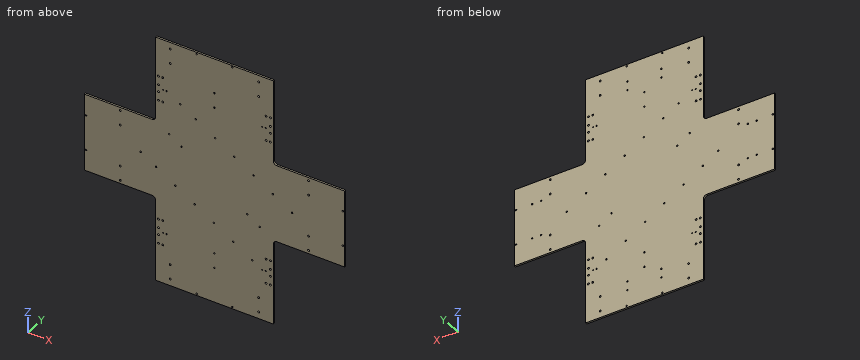
from build123d import *

# Parameters (mm, degrees)
BOSS_EXTRUDE1_DEPTH = 5
SKETCH2_R           = 2.125
CUT_EXTRUDE1_DEPTH  = 3
SKETCH4_R           = 2.6
SKETCH4_R_2         = 1.6
CUT_EXTRUDE3_DEPTH  = 10
SKETCH5_R           = 2.125
CUT_EXTRUDE4_DEPTH  = 10
FILLET1_R           = 10
SKETCH6_R           = 2.6
CUT_EXTRUDE5_DEPTH  = 10
SKETCH7_R           = 2.125
CUT_EXTRUDE6_DEPTH  = 10
SKETCH8_R           = 2.1
CUT_EXTRUDE7_DEPTH  = 10


with BuildPart() as part:
    # Sketch1 → Boss-Extrude1 (new body)
    with BuildSketch(Plane(origin=(0, 0, 0), x_dir=(1, 0, 0), z_dir=(0, 1, 0))):
        Polygon((165, 352), (-165, 352), (-165, 110), (-365, 110), (-365, -110), (-165, -110), (-165, -352), (165, -352), (165, -110), (365, -110), (365, 110), (165, 110), align=None)
    extrude(amount=BOSS_EXTRUDE1_DEPTH)

    # Sketch2 → Cut-Extrude1 (cut)
    with BuildSketch(Plane(origin=(0, 5, 0), x_dir=(1, 0, 0), z_dir=(0, 1, 0))):
        with Locations(Location((315, 49.5, 0), (0, 0, 270))):
            Circle(SKETCH2_R)
        with Locations(Location((290, 49.5, 0), (0, 0, 270))):
            Circle(SKETCH2_R)
        with Locations(Location((290, -49.5, 0), (0, 0, 90))):
            Circle(SKETCH2_R)
        with Locations(Location((315, -49.5, 0), (0, 0, 90))):
            Circle(SKETCH2_R)
        with Locations(Location((-315, -49.5, 0), (0, 0, 270))):
            Circle(SKETCH2_R)
        with Locations(Location((-290, -49.5, 0), (0, 0, 270))):
            Circle(SKETCH2_R)
        with Locations(Location((-290, 49.5, 0), (0, 0, 90))):
            Circle(SKETCH2_R)
        with Locations(Location((-315, 49.5, 0), (0, 0, 90))):
            Circle(SKETCH2_R)
        with Locations(Location((47.5, 302, 0), (0, 0, 270))):
            Circle(SKETCH2_R)
        with Locations(Location((47.5, 277, 0), (0, 0, 270))):
            Circle(SKETCH2_R)
        with Locations(Location((-47.5, 277, 0), (0, 0, 90))):
            Circle(SKETCH2_R)
        with Locations(Location((-47.5, 302, 0), (0, 0, 90))):
            Circle(SKETCH2_R)
        with Locations(Location((-47.5, -302, 0), (0, 0, 270))):
            Circle(SKETCH2_R)
        with Locations(Location((-47.5, -277, 0), (0, 0, 270))):
            Circle(SKETCH2_R)
        with Locations(Location((47.5, -277, 0), (0, 0, 90))):
            Circle(SKETCH2_R)
        with Locations(Location((47.5, -302, 0), (0, 0, 90))):
            Circle(SKETCH2_R)
    extrude(amount=-CUT_EXTRUDE1_DEPTH, mode=Mode.SUBTRACT)

    # Sketch4 → Cut-Extrude3 (cut)
    with BuildSketch(Plane(origin=(0, 5, 0), x_dir=(1, 0, 0), z_dir=(0, 1, 0))):
        with Locations(Location((-157, 172, 0), (0, 0, 270))):
            Circle(SKETCH4_R)
        with Locations(Location((-145, 172, 0), (0, 0, 270))):
            Circle(SKETCH4_R)
        with Locations(Location((-157, 197, 0), (0, 0, 270))):
            Circle(SKETCH4_R)
        with Locations(Location((-157, 217, 0), (0, 0, 270))):
            Circle(SKETCH4_R)
        with Locations(Location((-157, 242, 0), (0, 0, 270))):
            Circle(SKETCH4_R)
        with Locations(Location((-145, 242, 0), (0, 0, 270))):
            Circle(SKETCH4_R)
        with Locations(Location((145, 242, 0), (0, 0, 90))):
            Circle(SKETCH4_R)
        with Locations(Location((157, 242, 0), (0, 0, 90))):
            Circle(SKETCH4_R)
        with Locations(Location((157, 217, 0), (0, 0, 90))):
            Circle(SKETCH4_R)
        with Locations(Location((157, 197, 0), (0, 0, 90))):
            Circle(SKETCH4_R)
        with Locations(Location((145, 172, 0), (0, 0, 90))):
            Circle(SKETCH4_R)
        with Locations(Location((157, 172, 0), (0, 0, 90))):
            Circle(SKETCH4_R)
        with Locations(Location((157, -172, 0), (0, 0, 270))):
            Circle(SKETCH4_R)
        with Locations(Location((145, -172, 0), (0, 0, 270))):
            Circle(SKETCH4_R)
        with Locations(Location((157, -197, 0), (0, 0, 270))):
            Circle(SKETCH4_R)
        with Locations(Location((157, -217, 0), (0, 0, 270))):
            Circle(SKETCH4_R)
        with Locations(Location((157, -242, 0), (0, 0, 270))):
            Circle(SKETCH4_R)
        with Locations(Location((145, -242, 0), (0, 0, 270))):
            Circle(SKETCH4_R)
        with Locations(Location((-145, -242, 0), (0, 0, 90))):
            Circle(SKETCH4_R)
        with Locations(Location((-157, -242, 0), (0, 0, 90))):
            Circle(SKETCH4_R)
        with Locations(Location((-157, -217, 0), (0, 0, 90))):
            Circle(SKETCH4_R)
        with Locations(Location((-157, -197, 0), (0, 0, 90))):
            Circle(SKETCH4_R)
        with Locations(Location((-145, -172, 0), (0, 0, 90))):
            Circle(SKETCH4_R)
        with Locations(Location((-157, -172, 0), (0, 0, 90))):
            Circle(SKETCH4_R)
        with Locations(Location((144, -207, 0), (0, 0, 270))):
            Circle(SKETCH4_R_2)
        with Locations(Location((-144, -207, 0), (0, 0, 90))):
            Circle(SKETCH4_R_2)
        with Locations(Location((144, 207, 0), (0, 0, 90))):
            Circle(SKETCH4_R_2)
        with Locations(Location((-144, 207, 0), (0, 0, 270))):
            Circle(SKETCH4_R_2)
        with Locations(Location((134, -207, 0), (0, 0, 270))):
            Circle(SKETCH4_R_2)
        with Locations(Location((-134, -207, 0), (0, 0, 90))):
            Circle(SKETCH4_R_2)
        with Locations(Location((134, 207, 0), (0, 0, 90))):
            Circle(SKETCH4_R_2)
        with Locations(Location((-134, 207, 0), (0, 0, 270))):
            Circle(SKETCH4_R_2)
    extrude(amount=-CUT_EXTRUDE3_DEPTH, mode=Mode.SUBTRACT)

    # Sketch5 → Cut-Extrude4 (cut)
    with BuildSketch(Plane(origin=(0, 5, 0), x_dir=(1, 0, 0), z_dir=(0, 1, 0))):
        with Locations(Location((-50, 347, 0), (0, 0, 270))):
            Circle(SKETCH5_R)
        with Locations(Location((50, 347, 0), (0, 0, 270))):
            Circle(SKETCH5_R)
        with Locations(Location((50, -347, 0), (0, 0, 90))):
            Circle(SKETCH5_R)
        with Locations(Location((-50, -347, 0), (0, 0, 90))):
            Circle(SKETCH5_R)
        with Locations(Location((-360, 50, 0), (0, 0, 270))):
            Circle(SKETCH5_R)
        with Locations(Location((-360, -50, 0), (0, 0, 270))):
            Circle(SKETCH5_R)
        with Locations(Location((360, -50, 0), (0, 0, 90))):
            Circle(SKETCH5_R)
        with Locations(Location((360, 50, 0), (0, 0, 90))):
            Circle(SKETCH5_R)
    extrude(amount=-CUT_EXTRUDE4_DEPTH, mode=Mode.SUBTRACT)

    # Fillet1
    fillet1_edges = [part.edges().sort_by_distance(p)[0] for p in [
        (165, 2.5, -110),
        (165, 2.5, 110),
        (-165, 2.5, 110),
        (-165, 2.5, -110),
    ]]
    fillet(fillet1_edges, radius=FILLET1_R)

    # Sketch6 → Cut-Extrude5 (cut)
    with BuildSketch(Plane(origin=(0, 5, 0), x_dir=(1, 0, 0), z_dir=(0, 1, 0))):
        with Locations(Location((124, 333, 0), (0, 0, 270))):
            Circle(SKETCH6_R)
        with Locations(Location((124, 291.4, 0), (0, 0, 270))):
            Circle(SKETCH6_R)
        with Locations(Location((124, -291.4, 0), (0, 0, 90))):
            Circle(SKETCH6_R)
        with Locations(Location((124, -333, 0), (0, 0, 90))):
            Circle(SKETCH6_R)
        with Locations(Location((-124, -333, 0), (0, 0, 270))):
            Circle(SKETCH6_R)
        with Locations(Location((-124, -291.4, 0), (0, 0, 270))):
            Circle(SKETCH6_R)
        with Locations(Location((-124, 291.4, 0), (0, 0, 90))):
            Circle(SKETCH6_R)
        with Locations(Location((-124, 333, 0), (0, 0, 90))):
            Circle(SKETCH6_R)
        with Locations(Location((264, 101, 0), (0, 0, 270))):
            Circle(SKETCH6_R)
        with Locations(Location((264, 59.4, 0), (0, 0, 270))):
            Circle(SKETCH6_R)
        with Locations(Location((264, -59.4, 0), (0, 0, 90))):
            Circle(SKETCH6_R)
        with Locations(Location((264, -101, 0), (0, 0, 90))):
            Circle(SKETCH6_R)
        with Locations(Location((-264, -101, 0), (0, 0, 270))):
            Circle(SKETCH6_R)
        with Locations(Location((-264, -59.4, 0), (0, 0, 270))):
            Circle(SKETCH6_R)
        with Locations(Location((-264, 59.4, 0), (0, 0, 90))):
            Circle(SKETCH6_R)
        with Locations(Location((-264, 101, 0), (0, 0, 90))):
            Circle(SKETCH6_R)
    extrude(amount=-CUT_EXTRUDE5_DEPTH, mode=Mode.SUBTRACT)

    # Sketch7 → Cut-Extrude6 (cut)
    with BuildSketch(Plane(origin=(0, 5, 0), x_dir=(1, 0, 0), z_dir=(0, 1, 0))):
        with Locations(Location((-55.682048102, 90.197059371, 0), (0, 0, 270))):
            Circle(SKETCH7_R)
        with Locations(Location((-1.648904044, 123.553757998, 0), (0, 0, 270))):
            Circle(SKETCH7_R)
        with Locations(Location((52.384240013, 156.910456625, 0), (0, 0, 270))):
            Circle(SKETCH7_R)
        with Locations(Location((106.41738407, 190.267155252, 0), (0, 0, 270))):
            Circle(SKETCH7_R)
        with Locations(Location((-109.715192159, 56.840360744, 0), (0, 0, 270))):
            Circle(SKETCH7_R)
        with Locations(Location((-163.748336216, 23.483662117, 0), (0, 0, 270))):
            Circle(SKETCH7_R)
        with Locations(Location((-206.974851462, -3.201696784, 0), (0, 0, 270))):
            Circle(SKETCH7_R)
        with Locations(Location((-95.610755259, -183.595815527, 0), (0, 0, 90))):
            Circle(SKETCH7_R)
        with Locations(Location((-52.384240013, -156.910456625, 0), (0, 0, 90))):
            Circle(SKETCH7_R)
        with Locations(Location((1.648904044, -123.553757998, 0), (0, 0, 90))):
            Circle(SKETCH7_R)
        with Locations(Location((217.781480273, 9.87303651, 0), (0, 0, 90))):
            Circle(SKETCH7_R)
        with Locations(Location((163.748336216, -23.483662117, 0), (0, 0, 90))):
            Circle(SKETCH7_R)
        with Locations(Location((109.715192159, -56.840360744, 0), (0, 0, 90))):
            Circle(SKETCH7_R)
        with Locations(Location((55.682048102, -90.197059371, 0), (0, 0, 90))):
            Circle(SKETCH7_R)
    extrude(amount=-CUT_EXTRUDE6_DEPTH, mode=Mode.SUBTRACT)

    # Sketch8 → Cut-Extrude7 (cut)
    with BuildSketch(Plane(origin=(0, 5, 0), x_dir=(1, 0, 0), z_dir=(0, 1, 0))):
        with Locations(Location((-127.267902287, -85.585182493, 0), (0, 0, 270))):
            Circle(SKETCH8_R)
        with Locations(Location((-92.415590944, -62.147682754, 0), (0, 0, 270))):
            Circle(SKETCH8_R)
        with Locations(Location((92.415590944, 62.147682754, 0), (0, 0, 270))):
            Circle(SKETCH8_R)
        with Locations(Location((127.267902287, 85.585182493, 0), (0, 0, 270))):
            Circle(SKETCH8_R)
        with Locations(Location((0, 253, 0), (0, 0, 270))):
            Circle(SKETCH8_R)
        with Locations(Location((0, 211, 0), (0, 0, 270))):
            Circle(SKETCH8_R)
        with Locations(Location((0, -211, 0), (0, 0, 90))):
            Circle(SKETCH8_R)
        with Locations(Location((0, -253, 0), (0, 0, 90))):
            Circle(SKETCH8_R)
    extrude(amount=-CUT_EXTRUDE7_DEPTH, mode=Mode.SUBTRACT)


solid = part.part
The model under review builds one solid part; all positions refer to its coordinate system, in mm. Give positions to 0.01 mm unless a question says otherwise; leave off trailing zeros. Order: outer loops, then holes, each group sorted by start corner. A loop starts at its lowest first (then second) coordinate and runs counter-clockwise, first axis right, second up. Notation, with made-up numbers: M 60.25,73.25 L 105.25,73.25 A10 ccw 105.25,79.25 Z; hole C 81,41 d10. An arc over 180 degrees is marked long. Answer in a Markdown table with one row per item. Add a question column.
1. To check wall thickness, follow line 1 along Z through (x, y) = (264, 3.4); line 2 along Z through (x, y) = (-134, 2.15); line 3 along X through (y, z) = (3.1, -59.4). State the ranges of each line that lie inside material, in increasing order.
2. Add section B-B on y = 0.8. Count the separate pieces of the cut face and the enclosed holes in it, plus the area to 3 significant figures.
3. Add section A-A on x = -301. State the section outline as (y, z) points.
4. For pin 1 Ø4 at (x, z) = (163.75, 23.48) entering from +Y; pin 2 Ø1 at (y, z) = (4, 263) entering from -X; pin 3 Ø2 at (x, y) = (275, 2) entering from +Z; pin 4 Ø4 at (x, z) = (47.5, -302) entering from +Y, all flat-tipped, find the tip position at first contact; note any pin that passes through.
The answers:
| question | item | result |
|---|---|---|
| 1 | line 1 | -110 to -103.6, -98.4 to -62, -56.8 to 56.8, 62 to 98.4, 103.6 to 110 |
| 1 | line 2 | -352 to -208.6, -205.4 to 205.4, 208.6 to 352 |
| 1 | line 3 | -365 to -266.6, -261.4 to 261.4, 266.6 to 365 |
| 2 | separate pieces | 1 |
| 2 | enclosed holes | 78 |
| 2 | area | 319,000 mm2 |
| 3 | outline | M 0,-110 L 5,-110 L 5,110 L 0,110 Z |
| 4 | pin 1 | through |
| 4 | pin 2 | x = -165 |
| 4 | pin 3 | z = 110 |
| 4 | pin 4 | y = 2 |
